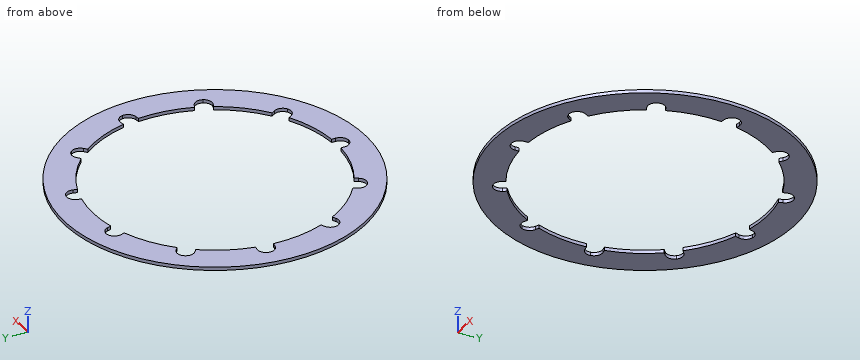
```python
from build123d import *

# Parameters (mm, degrees)
BOSS_EXTRUDE1_DEPTH      = 0.3175
BOSS_EXTRUDE1_DEPTH_BACK = 0.3175
SKETCH1_R                = 28.575
SKETCH1_R_2              = 23.114
SKETCH4_W                = 3.175
SKETCH4_H                = 6.35
CUT_EXTRUDE2_DEPTH       = 41.416141268
FILLET1_R                = 1.5875
CIRPATTERN1_COUNT        = 11
FILLET1_OF_CIRPATTERN1_R = 1.5875


with BuildPart() as part:
    # Sketch1 → Boss-Extrude1 (new, two sides: drawn at the far end of the back side and taken through both)
    with BuildSketch(Plane.XY.offset(-BOSS_EXTRUDE1_DEPTH_BACK)):
        Circle(SKETCH1_R)
        Circle(SKETCH1_R_2, mode=Mode.SUBTRACT)
    extrude(amount=BOSS_EXTRUDE1_DEPTH + BOSS_EXTRUDE1_DEPTH_BACK)

    # Sketch4 → Cut-Extrude2 (cut, through all)
    with BuildSketch(Plane.XY.offset(0.3175)):
        with Locations((0, -22.225)):
            Rectangle(SKETCH4_W, SKETCH4_H)
    cut_extrude2 = extrude(amount=-CUT_EXTRUDE2_DEPTH, mode=Mode.SUBTRACT)

    # Fillet1
    fillet1_edges = [part.edges().sort_by_distance(p)[0] for p in [
        (1.5875, -25.4, 0),
        (-1.5875, -25.4, 0),
    ]]
    fillet(fillet1_edges, radius=FILLET1_R - 0.0001)  # a hair under: the kernel refuses the full size

    # CirPattern1: Cut-Extrude2 ×11 about axis
    cirpattern1_axis = Axis((0, 0, 0), (0, 0, 1))
    for i in range(1, CIRPATTERN1_COUNT):
        add(cut_extrude2.rotate(cirpattern1_axis, i * 360 / CIRPATTERN1_COUNT), mode=Mode.SUBTRACT)

    # Fillet1 of CirPattern1
    fillet1_of_cirpattern1_edges = [part.edges().sort_by_distance(p)[0] for p in [
        (15.067766747, -20.509572436, 0),
        (12.39678678, -22.226107032, 0),
        (23.764124015, -9.107500538, 0),
        (22.445181349, -11.995582123, 0),
        (24.915539818, 5.186138431, 0),
        (25.36738943, 2.043455353, 0),
        (18.156447773, 17.833215091, 0),
        (20.235630604, 15.433710193, 0),
        (5.632811848, 24.818371964, 0),
        (8.679202039, 23.923871096, 0),
        (-8.679202039, 23.923871096, 0),
        (-5.632811848, 24.818371964, 0),
        (-20.235630604, 15.433710193, 0),
        (-18.156447773, 17.833215091, 0),
        (-25.36738943, 2.043455353, 0),
        (-24.915539818, 5.186138431, 0),
        (-22.445181349, -11.995582123, 0),
        (-23.764124015, -9.107500538, 0),
        (-12.39678678, -22.226107032, 0),
        (-15.067766747, -20.509572436, 0),
    ]]
    fillet(fillet1_of_cirpattern1_edges, radius=FILLET1_OF_CIRPATTERN1_R - 0.0001)  # a hair under: the kernel refuses the full size


solid = part.part
```
For this review, take the finished solid that the model builds, in its own axes (mm). Round coordinates to 2 decimals unless told otherwise and drop trailing zeros. Write each loop counter-clockwise with the first axis right and the second up, starting at its lowest first coordinate (ties: lowest second). Pieces come first, ordered by that corner, then holes. Notation, with made-up numbers: (21.25, 14) - (64.25, 14) arc R17 cw to (64.25, 25) - close; hole circle Ø1 at (-17.75, 21). An arc over 180 degrees is marked (long way). Answer as a JSON object with one key per item and string values.
1. We need section A-A on y = 0. Give the boundary of the cut face in (x, z) (1 decimal), then the cut area to 3 significant figures.
Response values:
{"outline": "(-28.6, -0.3) - (-23.1, -0.3) - (-23.1, 0.3) - (-28.6, 0.3) - close; (23.1, -0.3) - (28.6, -0.3) - (28.6, 0.3) - (23.1, 0.3) - close", "area": "6.94 mm2"}
2. To check wall thickness, follow line 1 along X through (y, z) = (-21, -0.05); line 2 along X through (y, z) = (4.5, -0.2); line 3 along Y through (x, z) = (-21, 0.2). State the ranges of each line that lie inside material, in increasing order.
Response values:
{"line 1": "x = -19.38 to -14.13, -11.62 to -9.66, 9.66 to 11.62, 14.13 to 19.38", "line 2": "x = -28.22 to -24.7, 24.7 to 28.22", "line 3": "y = -19.38 to -11.34, 9.66 to 19.38"}
3. We need section B-B on x = -6. Give the boundary of the cut face in (y, z), then the cut area to 3 significant figures.
Response values:
{"outline": "(-27.94, -0.32) - (-22.32, -0.32) - (-22.32, 0.32) - (-27.94, 0.32) - close; (24.27, -0.32) - (27.94, -0.32) - (27.94, 0.32) - (24.27, 0.32) - close", "area": "5.90 mm2"}
4. For pin 1 Ø12 at (x, y) = (-12, -2) entering from -Z; pin 2 Ø6 at (x, y) = (15.5, -15.5) entering from -Z, all flat-tipped, find the tip position at first contact; note any pin that passes through.
Response values:
{"pin 1": "passes through", "pin 2": "stops at z = -0.32"}
